from build123d import *

# Parameters (mm, degrees)
F0_W         = 300
F0_H         = 200
F0_R         = 15
F1_DEPTH     = 100
F2_R         = 10
F3_R         = 10
F4_R         = 10
F5_R         = 10
F6_T1_DEPTH  = 280
F6_T3_DEPTH  = 180
F6_T6_ANGLE  = 90
F6_T8_ANGLE  = 90
F6_T10_ANGLE = 90
F6_T12_ANGLE = 90
F7_T1_DEPTH  = 280
F7_T3_DEPTH  = 180
F7_T6_ANGLE  = 90
F7_T8_ANGLE  = 90
F7_T10_ANGLE = 90
F7_T12_ANGLE = 90


# Not quite as in the source:
# - a fillet or chamfer that OpenCascade refuses, or shapes differently, is made with other operations: its cross-section is extruded or revolved along the edge and cut away or added


with BuildPart() as f1:
    # F0 (on Top) → F1 (new body)
    with BuildSketch(Plane.XY):
        with Locations((-0.982619822, 16.5327907399)):
            Rectangle(F0_W, F0_H)
        with Locations((0, 100.119560957)):
            Circle(F0_R, mode=Mode.SUBTRACT)
    extrude(amount=F1_DEPTH)

    # F2
    f2_edges = [f1.edges().sort_by_distance(p)[0] for p in [
        (149.01738, 116.532791, 50),
    ]]
    fillet(f2_edges, radius=F2_R)

    # F3
    f3_edges = [f1.edges().sort_by_distance(p)[0] for p in [
        (-150.98262, 116.532791, 50),
    ]]
    fillet(f3_edges, radius=F3_R)

    # F4
    f4_edges = [f1.edges().sort_by_distance(p)[0] for p in [
        (149.01738, -83.467209, 50),
    ]]
    fillet(f4_edges, radius=F4_R)

    # F5
    f5_edges = [f1.edges().sort_by_distance(p)[0] for p in [
        (-150.98262, -83.467209, 50),
    ]]
    fillet(f5_edges, radius=F5_R)

    # F6: fillet of radius 10 on 9 edges, made by hand

    # F6_s2 → F6_t1 (cut)
    with BuildSketch(Plane.YZ.offset(-140.982619822)):
        with BuildLine():
            ThreePointArc((-83.4672092601, 90), (-80.538277072, 97.0710678119), (-73.4672092601, 100))
            Line((-73.4672092601, 100), (-83.4672092601, 100))
            Line((-83.4672092601, 100), (-83.4672092601, 90))
        make_face()
        with BuildLine():
            ThreePointArc((116.5327907399, 90), (113.6038585518, 97.0710678119), (106.5327907399, 100))
            Line((106.5327907399, 100), (116.5327907399, 100))
            Line((116.5327907399, 100), (116.5327907399, 90))
        make_face()
    extrude(amount=F6_T1_DEPTH, mode=Mode.SUBTRACT)

    # F6_s4 → F6_t3 (cut)
    with BuildSketch(Plane.XZ.offset(-106.5327907399)):
        with BuildLine():
            ThreePointArc((-150.982619822, 90), (-148.0536876339, 97.0710678119), (-140.982619822, 100))
            Line((-140.982619822, 100), (-150.982619822, 100))
            Line((-150.982619822, 100), (-150.982619822, 90))
        make_face()
        with BuildLine():
            ThreePointArc((149.017380178, 90), (146.0884479898, 97.0710678119), (139.017380178, 100))
            Line((139.017380178, 100), (149.017380178, 100))
            Line((149.017380178, 100), (149.017380178, 90))
        make_face()
    extrude(amount=F6_T3_DEPTH, mode=Mode.SUBTRACT)

    # F6_s5 → F6_t6 (revolve, cut)
    with BuildSketch(Plane.YZ.offset(-140.982619822)):
        with BuildLine():
            ThreePointArc((-83.4672092601, 90), (-80.538277072, 97.0710678119), (-73.4672092601, 100))
            Line((-73.4672092601, 100), (-83.4672092601, 100))
            Line((-83.4672092601, 100), (-83.4672092601, 90))
        make_face()
    revolve(axis=Axis((-140.982619822, -73.4672092601, 100), (0, 0, -1)), revolution_arc=F6_T6_ANGLE, mode=Mode.SUBTRACT)

    # F6_s7 → F6_t8 (revolve, cut)
    with BuildSketch(Plane.XZ.offset(73.4672092601)):
        with BuildLine():
            ThreePointArc((149.017380178, 90), (146.0884479898, 97.0710678119), (139.017380178, 100))
            Line((139.017380178, 100), (149.017380178, 100))
            Line((149.017380178, 100), (149.017380178, 90))
        make_face()
    revolve(axis=Axis((139.017380178, -73.4672092601, 100), (0, 0, -1)), revolution_arc=F6_T8_ANGLE, mode=Mode.SUBTRACT)

    # F6_s9 → F6_t10 (revolve, cut)
    with BuildSketch(Plane.YZ.offset(-140.982619822)):
        with BuildLine():
            ThreePointArc((116.5327907399, 90), (113.6038585518, 97.0710678119), (106.5327907399, 100))
            Line((106.5327907399, 100), (116.5327907399, 100))
            Line((116.5327907399, 100), (116.5327907399, 90))
        make_face()
    revolve(axis=Axis((-140.982619822, 106.5327907399, 100), (0, 0, 1)), revolution_arc=F6_T10_ANGLE, mode=Mode.SUBTRACT)

    # F6_s11 → F6_t12 (revolve, cut)
    with BuildSketch(Plane.XZ.offset(-106.5327907399)):
        with BuildLine():
            ThreePointArc((149.017380178, 90), (146.0884479898, 97.0710678119), (139.017380178, 100))
            Line((139.017380178, 100), (149.017380178, 100))
            Line((149.017380178, 100), (149.017380178, 90))
        make_face()
    revolve(axis=Axis((139.017380178, 106.5327907399, 100), (0, 0, 1)), revolution_arc=F6_T12_ANGLE, mode=Mode.SUBTRACT)

    # F6_s13 → F6_t14 (revolve, cut)
    with BuildSketch(Plane.XZ.offset(-100.119560957)):
        with BuildLine():
            ThreePointArc((15, 90), (17.9289321881, 97.0710678119), (25, 100))
            Line((25, 100), (15, 100))
            Line((15, 100), (15, 90))
        make_face()
    revolve(axis=Axis((0, 100.119560957, 100), (0, 0, 1)), mode=Mode.SUBTRACT)

    # F7: fillet of radius 10 on 9 edges, made by hand

    # F7_s2 → F7_t1 (cut)
    with BuildSketch(Plane.YZ.offset(-140.982619822)):
        with BuildLine():
            ThreePointArc((-73.4672092601, 0), (-80.538277072, 2.9289321881), (-83.4672092601, 10))
            Line((-83.4672092601, 10), (-83.4672092601, 0))
            Line((-83.4672092601, 0), (-73.4672092601, 0))
        make_face()
        with BuildLine():
            ThreePointArc((106.5327907399, 0), (113.6038585518, 2.9289321881), (116.5327907399, 10))
            Line((116.5327907399, 10), (116.5327907399, 0))
            Line((116.5327907399, 0), (106.5327907399, 0))
        make_face()
    extrude(amount=F7_T1_DEPTH, mode=Mode.SUBTRACT)

    # F7_s4 → F7_t3 (cut)
    with BuildSketch(Plane.XZ.offset(-106.5327907399)):
        with BuildLine():
            ThreePointArc((-140.982619822, 0), (-148.0536876339, 2.9289321881), (-150.982619822, 10))
            Line((-150.982619822, 10), (-150.982619822, 0))
            Line((-150.982619822, 0), (-140.982619822, 0))
        make_face()
        with BuildLine():
            ThreePointArc((139.017380178, 0), (146.0884479898, 2.9289321881), (149.017380178, 10))
            Line((149.017380178, 10), (149.017380178, 0))
            Line((149.017380178, 0), (139.017380178, 0))
        make_face()
    extrude(amount=F7_T3_DEPTH, mode=Mode.SUBTRACT)

    # F7_s5 → F7_t6 (revolve, cut)
    with BuildSketch(Plane.YZ.offset(-140.982619822)):
        with BuildLine():
            ThreePointArc((-73.4672092601, 0), (-80.538277072, 2.9289321881), (-83.4672092601, 10))
            Line((-83.4672092601, 10), (-83.4672092601, 0))
            Line((-83.4672092601, 0), (-73.4672092601, 0))
        make_face()
    revolve(axis=Axis((-140.982619822, -73.4672092601, 0), (0, 0, -1)), revolution_arc=F7_T6_ANGLE, mode=Mode.SUBTRACT)

    # F7_s7 → F7_t8 (revolve, cut)
    with BuildSketch(Plane.XZ.offset(73.4672092601)):
        with BuildLine():
            ThreePointArc((139.017380178, 0), (146.0884479898, 2.9289321881), (149.017380178, 10))
            Line((149.017380178, 10), (149.017380178, 0))
            Line((149.017380178, 0), (139.017380178, 0))
        make_face()
    revolve(axis=Axis((139.017380178, -73.4672092601, 0), (0, 0, -1)), revolution_arc=F7_T8_ANGLE, mode=Mode.SUBTRACT)

    # F7_s9 → F7_t10 (revolve, cut)
    with BuildSketch(Plane.YZ.offset(-140.982619822)):
        with BuildLine():
            ThreePointArc((106.5327907399, 0), (113.6038585518, 2.9289321881), (116.5327907399, 10))
            Line((116.5327907399, 10), (116.5327907399, 0))
            Line((116.5327907399, 0), (106.5327907399, 0))
        make_face()
    revolve(axis=Axis((-140.982619822, 106.5327907399, 0), (0, 0, 1)), revolution_arc=F7_T10_ANGLE, mode=Mode.SUBTRACT)

    # F7_s11 → F7_t12 (revolve, cut)
    with BuildSketch(Plane.XZ.offset(-106.5327907399)):
        with BuildLine():
            ThreePointArc((139.017380178, 0), (146.0884479898, 2.9289321881), (149.017380178, 10))
            Line((149.017380178, 10), (149.017380178, 0))
            Line((149.017380178, 0), (139.017380178, 0))
        make_face()
    revolve(axis=Axis((139.017380178, 106.5327907399, 0), (0, 0, 1)), revolution_arc=F7_T12_ANGLE, mode=Mode.SUBTRACT)

    # F7_s13 → F7_t14 (revolve, cut)
    with BuildSketch(Plane.XZ.offset(-100.119560957)):
        with BuildLine():
            ThreePointArc((25, 0), (17.9289321881, 2.9289321881), (15, 10))
            Line((15, 10), (15, 0))
            Line((15, 0), (25, 0))
        make_face()
    revolve(axis=Axis((0, 100.119560957, 0), (0, 0, 1)), mode=Mode.SUBTRACT)


solid = f1.part
Verification items for the finished model (mm, model axes). Round coordinates to 2 decimals unless told otherwise and drop trailing zeros. Loops run counter-clockwise (first coordinate to the right, second up) from the corner with the lowest first, then second, coordinate; pieces in that order, holes last. Notation, with made-up numbers: (-39.5, -30) - (-12.5, -30) arc R12 cw to (-12.5, -9) - close; hole circle Ø8 at (55, 19.25). An arc over 180 degrees is marked (long way). Answer in a Markdown table with one row per item. Add a question column.
Q1. Material ranges on line 1 (Y direction, x = 0, z = 58.5); line 2 (X direction, y = 106, z = 7); line 3 (Y direction, x = -1.5, z = 88), recorded low to high.
Q2. Section check A-A on x = 0. Enter the section's corners in (y, z).
Q3. Release check for a two-part mould opening along Y. For faces 1 (the face through (-147.976, 113.681, 50.56)), 2 (the face through (-3.252, 85.476, 49.44)), 3 (the face through (-150.983, 15, 49)) record: pulls with the +Y half, pulls with the -Y half, needs draft (parallel to the pull), parting line crosses it, or undercut.
Found:
| question | item | result |
|---|---|---|
| 1 | line 1 | y = -83.47 to 85.12, 115.12 to 116.53 |
| 1 | line 2 | x = -150.52 to -14.3, 14.3 to 148.56 |
| 1 | line 3 | y = -83.47 to 85.19, 115.04 to 116.53 |
| 2 | outline | (-83.47, 10) arc R10 ccw to (-73.47, 0) - (75.12, 0) arc R10 ccw to (85.12, 10) - (85.12, 90) arc R10 ccw to (75.12, 100) - (-73.47, 100) arc R10 ccw to (-83.47, 90) - close; (115.12, 10) arc R10 ccw to (115.83, 6.31) arc R10 ccw to (116.53, 10) - (116.53, 90) arc R10 ccw to (115.83, 93.69) arc R10 ccw to (115.12, 90) - close |
| 3 | face 1 | pulls with the +Y half |
| 3 | face 2 | undercut |
| 3 | face 3 | needs draft |
